from build123d import *

# Parameters (mm, degrees)
Y_KSEKLIK_EKSTR_ZYON1_DEPTH = 25
IZIM2_R                     = 2
KES_EKSTR_ZYON1_DEPTH       = 25
IZIM3_R                     = 5.5
IZIM3_W                     = 8
IZIM3_H                     = 30
KES_EKSTR_ZYON2_DEPTH       = 10
CUT_EXTRUDE8_DEPTH          = 7.5
RADYUS1_R                   = 4
FILLET1_R                   = 12.5


with BuildPart() as part:
    # Çizim1 → Yükseklik-Ekstrüzyon1 (new body)
    with BuildSketch(Plane.XY):
        Polygon((-2.5, 48), (-12.5, 48), (-12.5, 90), (-7.5, 90), (-7.5, 59), (7.5, 59), (7.5, 90), (12.5, 90), (12.5, 48), (2.5, 48), (2.5, -87.5), (-2.5, -87.5), align=None)
    extrude(amount=Y_KSEKLIK_EKSTR_ZYON1_DEPTH)

    # Çizim2 → Kes-Ekstrüzyon1 (cut)
    with BuildSketch(Plane.ZY.offset(12.5)):
        with Locations((12.5, 77.5)):
            Circle(IZIM2_R)
    extrude(amount=-KES_EKSTR_ZYON1_DEPTH, mode=Mode.SUBTRACT)

    # Çizim3 → Kes-Ekstrüzyon2 (cut)
    with BuildSketch(Plane.ZY.offset(2.5)):
        with Locations((12.5, -72.5)):
            Circle(IZIM3_R)
        with Locations((12.5, 22.5)):
            Rectangle(IZIM3_W, IZIM3_H)
        with Locations((12.5, -32.5)):
            Rectangle(IZIM3_W, IZIM3_H)
    extrude(amount=-KES_EKSTR_ZYON2_DEPTH, mode=Mode.SUBTRACT)

    # Sketch2 → Cut-Extrude8 (cut, symmetric)
    with BuildSketch(Plane(origin=(0, 0, 0), x_dir=(0, 0, -1), z_dir=(1, 0, 0))):
        Polygon((-12.5, 63), (-25.5, 51), (-25.5, 65), (0.5, 65), (0.5, 51), align=None)
    extrude(amount=CUT_EXTRUDE8_DEPTH, both=True, mode=Mode.SUBTRACT)

    # Radyus1
    radyus1_edges = [part.edges().sort_by_distance(p)[0] for p in [
        (-10, 90, 25),
        (10, 90, 25),
        (10, 90, 0),
        (-10, 90, 0),
        (0, 7.5, 16.5),
        (0, 37.5, 16.5),
        (0, 7.5, 8.5),
        (0, 37.5, 8.5),
        (0, -47.5, 16.5),
        (0, -47.5, 8.5),
        (0, -17.5, 16.5),
        (0, -17.5, 8.5),
        (0, 59, 16.833333333),
        (0, 59, 8.166666667),
        (12.5, 48, 12.5),
        (-12.5, 48, 12.5),
    ]]
    fillet(radyus1_edges, radius=RADYUS1_R - 0.0001)  # a hair under: the kernel refuses the full size

    # Fillet1
    fillet1_edges = [part.edges().sort_by_distance(p)[0] for p in [
        (0, -87.5, 0),
        (0, -87.5, 25),
    ]]
    fillet(fillet1_edges, radius=FILLET1_R - 0.0001)  # a hair under: the kernel refuses the full size


solid = part.part
Work out the finished part from the listing and answer in its coordinate system (mm). A direction names the side the tool comes from. Give positions to 0.01 mm unless a question says otherwise; leave off trailing zeros. Order: outer loops, then holes, each group sorted by start corner. A loop starts at its lowest first (then second) coordinate and runs counter-clockwise, first axis right, second up. Notation, with made-up numbers: (26.25, 23) -> (31.25, 23) arc R31 ccw to (31.25, 51) -> close; hole circle Ø8 at (-26.75, 45.5). An arc over 180 degrees is marked (long way). Answer as a JSON object with one key per item and string values. Group by question number.
1. Section D-D on z = 23.25 is taken. Determine the outline of the cut face in (x, y).
2. Section C-C on x = 11 is taken. Determine the outline of the cut face in (y, z).
3. Section A-A on y = -72.5 is taken. Determine the outline of the cut face in (x, z).
4. Consider line 1 along Y through (x, z) = (0.1, 12.5); line 2 along X through (y, z) = (57, 5); line 3 along Y through (x, z) = (-0.75, 9). Determine where each line is inside the solid, lowest interval first. Write a range as [from, to].
5. Flat-ended cylindrical pins translate along their axes: pin 1 Ø3 at (x, y) = (4.5, -33) entering from -Z; pin 2 Ø7.5 at (y, z) = (-10, 7) entering from -X; pin 3 Ø5 at (x, z) = (-5.5, 20) entering from -Y; pin 4 Ø5 at (x, z) = (-3, 6.5) entering from +Y. Find the tip coordinate at first contact, or state that the pin passes through.
6. The mould has two halves that part along X. Classify faces 1 (the flat face through (2.5, -19, 7)), 2 (the cylindrical face through (0.035, 8.641, 15.297)), 3 (the flat face through (0.105, 54.655, 3.46)): released by +X, released by -X, zero draft, split by the parting line, or undercut.
7. A tool of negligible diameter and unlimited length cuts with its end or side. For faces 4 (the flat face through (-10, 90, 12)), 5 (the flat face through (6, 48, 12)), 6 (the cylindrical face through (0.035, -46.359, 15.297)), from which of +Z, -Z, +X, -X, +Y, -Y can it reach the whole face along a straight path? Write none if from no direction.
8. Section B-B on y = 77.5 is taken. Determine the outline of the cut face in (x, z).
Result sheet:
{
 "1": {"outline": "(-12.5, 52) arc R4 ccw to (-8.5, 48) -> (-2.5, 48) -> (-2.5, -81.38) -> (2.5, -81.38) -> (2.5, 48) -> (8.5, 48) arc R4 ccw to (12.5, 52) -> (12.5, 89.31) -> (7.5, 89.31) -> (7.5, 53.08) -> (-7.5, 53.08) -> (-7.5, 89.31) -> (-12.5, 89.31) -> close"},
 "2": {"outline": "(48.88, 0) -> (86, 0) arc R4 ccw to (90, 4) -> (90, 21) arc R4 ccw to (86, 25) -> (48.88, 25) -> close; hole circle Ø4 at (77.5, 12.5)"},
 "3": {"outline": "(-2.5, 0) -> (2.5, 0) -> (2.5, 7) -> (-2.5, 7) -> close; (-2.5, 18) -> (2.5, 18) -> (2.5, 25) -> (-2.5, 25) -> close"},
 "4": {"line 1": "y = [-87.5, -78], [-67, -47.5], [-17.5, 7.5], [37.5, 59]", "line 2": "x = [-12.5, -7.5], [7.5, 12.5]", "line 3": "y = [-87, -76.74], [-68.26, -45.44], [-19.56, 9.56], [35.44, 58.93]"},
 "5": {"pin 1": "passes through", "pin 2": "stops at x = -2.5", "pin 3": "stops at y = 48", "pin 4": "stops at y = 58.93"},
 "6": {"face 1": "released by +X", "face 2": "zero draft", "face 3": "undercut"},
 "7": {"face 4": "+Z, -Z, +X, -X, +Y", "face 5": "+Z, -Z, +X, -Y", "face 6": "+X, -X"},
 "8": {"outline": "(-12.5, 0) -> (-7.5, 0) -> (-7.5, 10.5) -> (-12.5, 10.5) -> close; (-12.5, 14.5) -> (-7.5, 14.5) -> (-7.5, 25) -> (-12.5, 25) -> close; (7.5, 0) -> (12.5, 0) -> (12.5, 10.5) -> (7.5, 10.5) -> close; (7.5, 14.5) -> (12.5, 14.5) -> (12.5, 25) -> (7.5, 25) -> close"}
}
